Work out the finished part from the listing and answer in its coordinate system (mm). Face numbers are marked on the shaded views. Coordinates: 2 decimals unless noted, no trailing zeros. Write each loop counter-clockwise with the first axis right and the second up, starting at its lowest first coordinate (ties: lowest second). Pieces come first, ordered by that corner, then holes. Notation, with made-up numbers: (20, 46.5) - (43, 46.5) arc R24 ccw to (43, 69.5) - close; hole circle Ø6 at (-23.5, -26.5). An arc over 180 degrees is marked (long way). Use a Markdown table: item, result. Add a question column.
(1) Given pin 1 Ø1.6 at (y, z) = (5.66, 17.66) entering from -X; pin 2 Ø2 at (y, z) = (0, 20) entering from -X; pin 3 Ø4.5 at (y, z) = (8, 12) entering from -X; pin 4 Ø3.5 at (y, z) = (0, 20) entering from +X, each flat-ended and moving along its own axis, determine where each tip first touches the part or whether it passes through.
(2) Find the intervals of material crossed by line 1 (Y direction, x = -1.5, z = 11.75); line 2 (Y direction, x = -8, z = 12.5); line 3 (Z direction, x = -6, y = -6.25), in increasing order. Write a range as from..to.
(3) The part is cut by section B-B, the plane x = 6.25. State how many separate pieces and enclosed holes the cut face has, then the cut area to 3 significant figures.
(4) For a pull along Z with two mould halves and no side action, classify the marked faces 1, 2 and 3 as released by +Z, released by -Z, zero draft, split by the parting line, or undercut.
(5) The part is cut by section A-A, the plane x = 2.75. Give the vertices of the cut face in (y, z).
from build123d import *

# Parameters (mm, degrees)
F0_W     = 20
F0_H     = 24
F1_DEPTH = 24
F2_R     = 4
F3_DEPTH = 20.001
F5_D     = 2.7051
F5_DEPTH = 6
F5_TIP   = 0.8126940303
F7_D     = 2.7051
F7_DEPTH = 6
F7_TIP   = 0.8126940303
F8_R     = 1
F9_SIZE  = 0.5


with BuildPart() as f1:
    # F0 (on Top) → F1 (new body)
    with BuildSketch(Plane.XY):
        Rectangle(F0_W, F0_H)
    extrude(amount=F1_DEPTH)

    # F2 (on face) → F3 (cut, through all)
    with BuildSketch(Plane.YZ.offset(10)):
        with Locations((0, 12)):
            Circle(F2_R)
    extrude(amount=-F3_DEPTH, mode=Mode.SUBTRACT)

    # F5
    with Locations(Plane.YZ.offset(10)):
        with Locations((0, 20), (5.6568542495, 17.6568542495), (8, 12), (5.6568542495, 6.3431457505), (0, 4), (-5.6568542495, 6.3431457505), (-8, 12), (-5.6568542495, 17.6568542495)):
            Hole(F5_D / 2, depth=F5_DEPTH)
            with Locations((0, 0, -(F5_DEPTH + F5_TIP / 2))):  # 118° drill point
                Cone(0, F5_D / 2, F5_TIP, mode=Mode.SUBTRACT)

    # F7
    with Locations(Plane(origin=(-10, 0, 0), x_dir=(0, -1, 0), z_dir=(-1, 0, 0))):
        with Locations((0, 20), (5.6568542495, 17.6568542495), (8, 12), (5.6568542495, 6.3431457505), (0, 4), (-5.6568542495, 6.3431457505), (-8, 12), (-5.6568542495, 17.6568542495)):
            Hole(F7_D / 2, depth=F7_DEPTH)
            with Locations((0, 0, -(F7_DEPTH + F7_TIP / 2))):  # 118° drill point
                Cone(0, F7_D / 2, F7_TIP, mode=Mode.SUBTRACT)

    # F8
    f8_edges = [f1.edges().sort_by_distance(p)[0] for p in [
        (0, -12, 24),
        (10, 0, 24),
        (0, 12, 24),
        (-10, 0, 24),
        (-10, -12, 12),
        (10, -12, 12),
        (0, -12, 0),
        (10, 12, 12),
        (-10, 12, 12),
        (0, 12, 0),
        (10, 0, 0),
        (-10, 0, 0),
    ]]
    fillet(f8_edges, radius=F8_R)

    # F9
    f9_edges = [f1.edges().sort_by_distance(p)[0] for p in [
        (10, -4, 12),
        (-10, -4, 12),
        (-10, 7.009404, 17.656854),
        (-10, 1.35255, 20),
        (-10, -4.304304, 17.656854),
        (-10, 9.35255, 12),
        (-10, 7.009404, 6.343146),
        (-10, -6.64745, 12),
        (-10, 1.35255, 4),
        (-10, -4.304304, 6.343146),
        (10, -7.009404, 17.656854),
        (10, -1.35255, 20),
        (10, 4.304304, 17.656854),
        (10, -9.35255, 12),
        (10, -7.009404, 6.343146),
        (10, 6.64745, 12),
        (10, -1.35255, 4),
        (10, 4.304304, 6.343146),
    ]]
    chamfer(f9_edges, length=F9_SIZE)


solid = f1.part
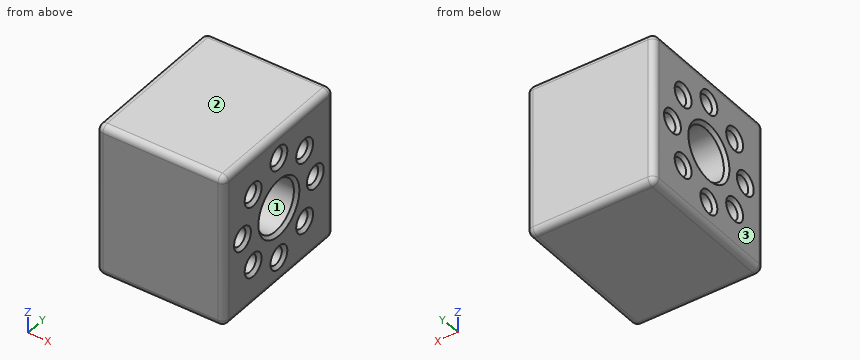
Model answer:
| question | item | result |
|---|---|---|
| 1 | pin 1 | x = -3.67 |
| 1 | pin 2 | x = -3.79 |
| 1 | pin 3 | x = -10 |
| 1 | pin 4 | x = 9.9 |
| 2 | line 1 | -12..-3.99, 3.99..12 |
| 2 | line 2 | -12..-9.26, -6.74..-3.97, 3.97..6.74, 9.26..12 |
| 2 | line 3 | 0..5.13, 7.56..16.44, 18.87..24 |
| 3 | separate pieces | 1 |
| 3 | enclosed holes | 9 |
| 3 | area | 479 mm^2 |
| 4 | face 1 | undercut |
| 4 | face 2 | released by +Z |
| 4 | face 3 | zero draft |
| 5 | outline | (-12, 1) arc R1 ccw to (-11, 0) - (11, 0) arc R1 ccw to (12, 1) - (12, 23) arc R1 ccw to (11, 24) - (-11, 24) arc R1 ccw to (-12, 23) - close; hole circle Ø8 at (0, 12) |
